Geometry: see drawing. Coordinates: mm, zero at the bounding-box minimum. A direction names the side the tool comes from. Give positions to 0.01 mm unless a question says otherwise; leave off trailing zeros. Write each loop counter-clockwise with the first axis right and the second up, starting at its lowest first coordinate (ties: lowest second). Pieces come first, ordered by that corner, then holes. Notation, with made-up numbers: (26.25, 3.5) - (50.25, 3.5) arc R21 ccw to (50.25, 18.5) - close; hole circle Ø6 at (-13.75, -18.75). An arc over 180 degrees is marked (long way). Use a Markdown table: item, result. Add a question column.
1. Set-up query: the marked faces 4, 5 and 6. Return all of +Z, -Z, +X, -X, +Y, -Y with unobstructed straight access to the full face (end or side cutting, diameter ignored); none if empty.
2. Mould query, pull axis Z, two halves, no side actions, for the marked faces 1, 2 and 3. Classes: released by +Z, released by -Z, zero draft, split by the parting line, or undercut.
3. Section query B-B, the plane x = 8. Return loops of the section in (y, z).
4. Pin query (flat end, axial travel): pin 1 (1 mm diameter, centred on x = 21, y = 2.5, fed in from -Z); pin 2 (6 mm diameter, centred on y = 4.5, z = 68.5, fed in from +X); pin 3 (5 mm diameter, centred on x = 81.5, y = 7, fed in from -Z) (1 decimal); pin 4 (3 mm diameter, centred on x = 68, z = 27, fed in from +Y). Return the tip coordinate at first contact, or that it passes through.
5. Section query D-D, the plane z = 63. Return loops of the section in (x, y).
6. Material intervals for probe 1 along X at (y, z) = (0.85, 70); probe 2 along Z at (x, y) = (25, 6.5) (1 decimal); probe 3 along X at (y, z) = (2.25, 29), sorted ascending.
7. Section query A-A, the plane y = 7.5. Return loops of the section in (x, z) (1 decimal), plus the area to 3 significant figures.
8. Section query C-C, the plane z = 36.5. Return loops of the section in (x, y), plus the area to 3 significant figures.
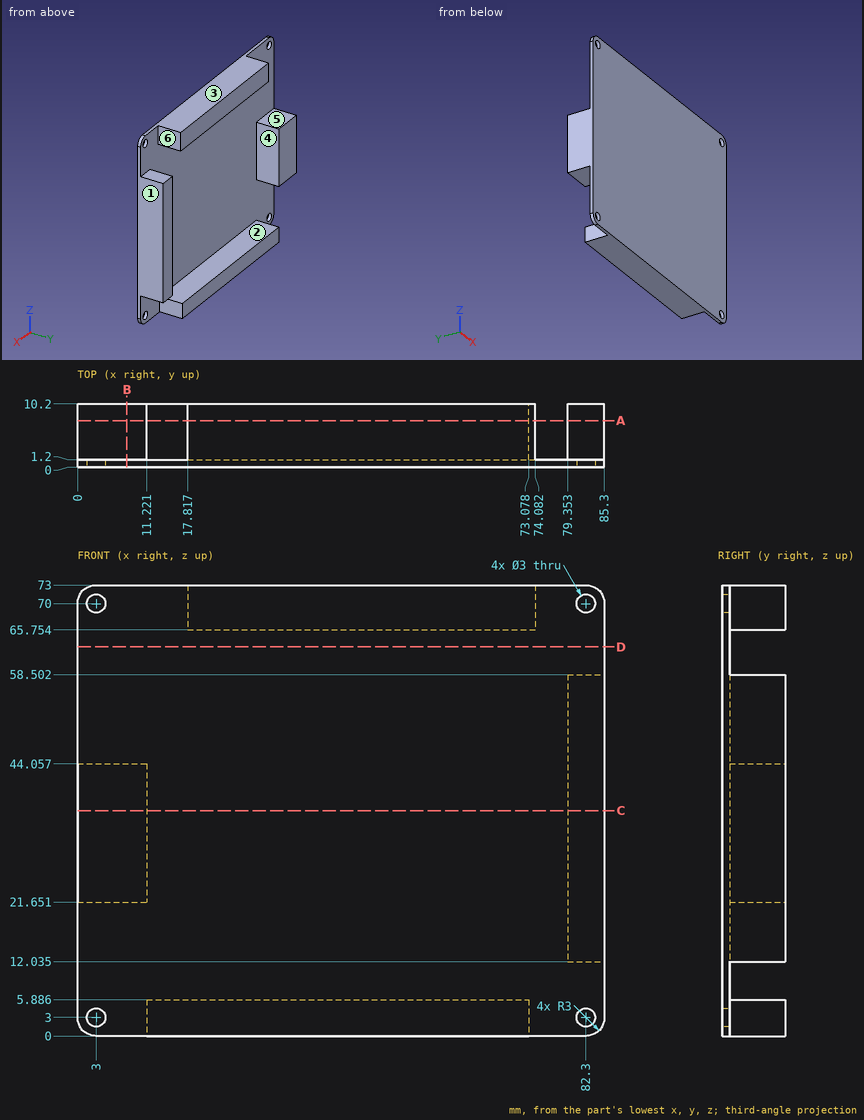
Result sheet:
| question | item | result |
|---|---|---|
| 1 | face 4 | +Z, +Y |
| 1 | face 5 | +Z, -X, +Y |
| 1 | face 6 | +Z, -Z, +X, +Y |
| 2 | face 1 | zero draft |
| 2 | face 2 | undercut |
| 2 | face 3 | released by +Z |
| 3 | outline | (0, 0) - (1.2, 0) - (1.2, 21.65) - (10.2, 21.65) - (10.2, 44.06) - (1.2, 44.06) - (1.2, 73) - (0, 73) - close |
| 4 | pin 1 | stops at z = 0 |
| 4 | pin 2 | stops at x = 74.08 |
| 4 | pin 3 | stops at z = 12 |
| 4 | pin 4 | stops at y = 1.2 |
| 5 | outline | (0, 0) - (85.3, 0) - (85.3, 1.2) - (0, 1.2) - close |
| 6 | probe 1 | x = 0 to 1.5, 4.5 to 80.8, 83.8 to 85.3 |
| 6 | probe 2 | z = 0 to 5.9, 65.8 to 73 |
| 6 | probe 3 | x = 0 to 11.22, 79.35 to 85.3 |
| 7 | outline | (0, 21.7) - (11.2, 21.7) - (11.2, 44.1) - (0, 44.1) - close; (11.2, 0) - (73.1, 0) - (73.1, 5.9) - (11.2, 5.9) - close; (17.8, 65.8) - (74.1, 65.8) - (74.1, 73) - (17.8, 73) - close; (79.4, 12) - (85.3, 12) - (85.3, 58.5) - (79.4, 58.5) - close |
| 7 | area | 1,300 mm² |
| 8 | outline | (0, 0) - (85.3, 0) - (85.3, 10.2) - (79.35, 10.2) - (79.35, 1.2) - (11.22, 1.2) - (11.22, 10.2) - (0, 10.2) - close |
| 8 | area | 257 mm² |
